Check sheet for the modelled part. Datum: model origin and axes. Units: mm. A direction names the side the tool comes from. Round coordinates to 2 decimals unless told otherwise and drop trailing zeros. Order: outer loops, then holes, each group sorted by start corner. A loop starts at its lowest first (then second) coordinate and runs counter-clockwise, first axis right, second up. Notation, with made-up numbers: (22, 28.5) -> (63, 28.5) arc R14 ccw to (63, 41.5) -> close; hole circle Ø1 at (2.5, 70.25). An arc over 180 degrees is marked (long way). Answer as CSV lines item,"result". Start each with the question number.
from build123d import *

# Parameters (mm, degrees)
SM_BASE_FLANGE_1_DEPTH = 2
OTHER_START            = -4.5
OTHER_3_DEPTH          = 20
OTHER_3_2_OUTLINE_W    = 2
OTHER_3_2_OUTLINE_H    = 24
OTHER_3_2_DEPTH        = 20
OTHER_START_2          = 5.5
OTHER_3_3_OUTLINE_W    = 2
OTHER_3_3_OUTLINE_H    = 15
OTHER_3_3_OUTLINE_H_2  = 9
OTHER_3_3_DEPTH        = 10
OTHER_START_3          = 4.5
OTHER_3_4_OUTLINE_W    = 2
OTHER_3_4_OUTLINE_H    = 15
OTHER_3_4_DEPTH        = 1
OTHER_4_DEPTH          = 20
OTHER_4_2_DEPTH        = 9
OTHER_4_3_DEPTH        = 11
OTHER_4_4_DEPTH        = 9
SKETCH_10_R            = 1.6
CUT_EXTRUDE_1_DEPTH    = 10
SKETCH_11_R            = 1.6
CUT_EXTRUDE_2_DEPTH    = 10
SKETCH_13_R            = 1.6
CUT_EXTRUDE_3_DEPTH    = 87
CUT_EXTRUDE_4_DEPTH    = 87
SKETCH_15_R            = 1.6
CUT_EXTRUDE_5_DEPTH    = 87
FILLET_1_R             = 3
FILLET_2_R             = 2


# Read off the part's stored shape, not the designer's step: 绘制的折弯3, 绘制的折弯4
# Sheet-metal steps are written as plain solids
with BuildPart() as part:
    # Sketch 1 → 基体-法兰1 (new body)
    with BuildSketch(Plane(origin=(0, 0, 0), x_dir=(1, 0, 0), z_dir=(0, 1, 0))):
        Polygon((-16, -15.5), (16, -15.5), (73, -15.5), (73, -4.5), (58, -4.5), (58, 4.5), (34, 4.5), (34, -5.5), (25, -5.5), (25, 4.5), (16, 4.5), (16, 15.5), (-16, 15.5), align=None)
    extrude(amount=-SM_BASE_FLANGE_1_DEPTH)

    # Other 3 outline → Other 3 (cut)
    with BuildSketch(Plane.XY.offset(OTHER_START)):
        with BuildLine():
            ThreePointArc((18.929203673, 0), (20.661254481, -0.550510257), (21.757630798, -2))
            Line((21.757630798, -2), (73, -2))
            Line((73, -2), (73, 0))
            Line((73, 0), (18.929203673, 0))
        make_face()
    extrude(amount=OTHER_3_DEPTH, mode=Mode.SUBTRACT)

    # Other 3 2 outline → Other 3 2 (add)
    with BuildSketch(Plane.XY.offset(OTHER_START)):
        with Locations((20.929203673, -26.929203673)):
            Rectangle(OTHER_3_2_OUTLINE_W, OTHER_3_2_OUTLINE_H)
        with BuildLine():
            Line((19.929203673, -3), (19.929203673, -5.929203673))
            Line((19.929203673, -5.929203673), (21.929203673, -5.929203673))
            Line((21.929203673, -5.929203673), (21.929203673, -3))
            ThreePointArc((21.929203673, -3), (21.885999352, -2.492694064), (21.757630798, -2))
            Line((21.757630798, -2), (18.929203673, -2))
            ThreePointArc((18.929203673, -2), (19.636310454, -2.292893219), (19.929203673, -3))
        make_face()
    extrude(amount=OTHER_3_2_DEPTH)

    # Other 3 3 outline → Other 3 3 (add)
    with BuildSketch(Plane.XY.offset(OTHER_START_2)):
        with Locations((20.929203673, -46.429203673)):
            Rectangle(OTHER_3_3_OUTLINE_W, OTHER_3_3_OUTLINE_H)
        with Locations((20.929203673, -10.429203673)):
            Rectangle(OTHER_3_3_OUTLINE_W, OTHER_3_3_OUTLINE_H_2)
    extrude(amount=OTHER_3_3_DEPTH)

    # Other 3 4 outline → Other 3 4 (add)
    with BuildSketch(Plane.XY.offset(OTHER_START_3)):
        with Locations((20.929203673, -46.429203673)):
            Rectangle(OTHER_3_4_OUTLINE_W, OTHER_3_4_OUTLINE_H)
    extrude(amount=OTHER_3_4_DEPTH)

    # Other 4 outline → Other 4 (cut)
    with BuildSketch(Plane.XY.offset(OTHER_START)):
        with BuildLine():
            Line((19.929203673, -40.186834471), (19.929203673, -53.929203673))
            Line((19.929203673, -53.929203673), (21.929203673, -53.929203673))
            Line((21.929203673, -53.929203673), (21.929203673, -37.358407346))
            ThreePointArc((21.929203673, -37.358407346), (21.378693416, -39.090458154), (19.929203673, -40.186834471))
        make_face()
    extrude(amount=OTHER_4_DEPTH, mode=Mode.SUBTRACT)

    # Other 4 2 outline → Other 4 2 (cut)
    with BuildSketch(Plane.XY.offset(OTHER_START)):
        Polygon((19.929203673, -38.929203673), (20.5, -38.929203673), (19.929203673, -38.358407347), align=None)
    extrude(amount=OTHER_4_2_DEPTH, mode=Mode.SUBTRACT)

    # Other 4 3 outline → Other 4 3 (add)
    with BuildSketch(Plane.XY.offset(OTHER_START_3)):
        with BuildLine():
            ThreePointArc((18.929203673, -40.358407346), (19.436509609, -40.315203025), (19.929203673, -40.186834471))
            Line((19.929203673, -40.186834471), (19.929203673, -37.358407346))
            ThreePointArc((19.929203673, -37.358407346), (19.636310454, -38.065514128), (18.929203673, -38.358407346))
            Line((18.929203673, -38.358407346), (5.5, -38.358407346))
            Line((5.5, -38.358407346), (5.5, -40.358407346))
            Line((5.5, -40.358407346), (18.929203673, -40.358407346))
        make_face()
    extrude(amount=OTHER_4_3_DEPTH)

    # Other 4 4 outline → Other 4 4 (add)
    with BuildSketch(Plane.XY.offset(OTHER_START)):
        with BuildLine():
            Line((20.5, -38.929203673), (21.050524017, -39.47972769))
            ThreePointArc((21.050524017, -39.47972769), (21.283955222, -39.217209419), (21.485098605, -38.929203673))
            Line((21.485098605, -38.929203673), (20.5, -38.929203673))
        make_face()
        with BuildLine():
            Line((19.636310454, -38.065514128), (19.929203673, -38.358407347))
            Line((19.929203673, -38.358407347), (19.929203673, -37.358407346))
            ThreePointArc((19.929203673, -37.358407346), (19.853083206, -37.741090779), (19.636310454, -38.065514128))
        make_face()
    extrude(amount=OTHER_4_4_DEPTH)

    # 草图10 → 切除-拉伸1 (cut)
    with BuildSketch(Plane(origin=(0, 0, 0), x_dir=(1, 0, 0), z_dir=(0, 1, 0))):
        with Locations(Location((-12.5, 12.5, 0), (0, 0, 270))):
            Circle(SKETCH_10_R)
        with Locations(Location((12.5, 12.5, 0), (0, 0, 270))):
            Circle(SKETCH_10_R)
    extrude(amount=-CUT_EXTRUDE_1_DEPTH, mode=Mode.SUBTRACT)

    # 草图11 → 切除-拉伸2 (cut)
    with BuildSketch(Plane(origin=(0, 0, 0), x_dir=(1, 0, 0), z_dir=(0, 1, 0))):
        with Locations(Location((-12.8, -12.3, 0), (0, 0, 270))):
            Circle(SKETCH_11_R)
        with Locations(Location((-4.5, -12.3, 0), (0, 0, 270))):
            Circle(SKETCH_11_R)
    extrude(amount=-CUT_EXTRUDE_2_DEPTH, mode=Mode.SUBTRACT)

    # 草图13 → 切除-拉伸3 (cut)
    with BuildSketch(Plane(origin=(0, -40.358407346, 0), x_dir=(-1, 0, 0), z_dir=(0, -1, 0))):
        with Locations(Location((-8.5, -10, 0), (0, 0, 180))):
            Circle(SKETCH_13_R)
        with Locations(Location((-15.5, -10, 0), (0, 0, 180))):
            Circle(SKETCH_13_R)
    extrude(amount=-CUT_EXTRUDE_3_DEPTH, mode=Mode.SUBTRACT)

    # 草图14 → 切除-拉伸4 (cut)
    with BuildSketch(Plane(origin=(21.929203673, 0, 0), x_dir=(0, 0, -1), z_dir=(1, 0, 0))):
        with BuildLine():
            Line((-10.3, -19.758407346), (-10.3, -20.179203673))
            Line((-10.3, -20.179203673), (-10.3, -21.358407346))
            ThreePointArc((-10.3, -21.358407346), (-9.16862915, -20.889778196), (-8.7, -19.758407346))
            ThreePointArc((-8.7, -19.758407346), (-9.16862915, -18.627036497), (-10.3, -18.158407346))
            Line((-10.3, -18.158407346), (-10.3, -19.758407346))
        make_face()
        with BuildLine():
            ThreePointArc((-10.3, -18.158407346), (-11.571470433, -18.78713862), (-11.843674335, -20.179203673))
            Line((-11.843674335, -20.179203673), (-10.3, -20.179203673))
            Line((-10.3, -20.179203673), (-10.3, -19.758407346))
            Line((-10.3, -19.758407346), (-10.3, -18.158407346))
        make_face()
        with BuildLine():
            Line((-10.3, -20.179203673), (-11.843674335, -20.179203673))
            ThreePointArc((-11.843674335, -20.179203673), (-11.271268726, -21.029877779), (-10.3, -21.358407346))
            Line((-10.3, -21.358407346), (-10.3, -20.179203673))
        make_face()
        with BuildLine():
            ThreePointArc((-8.7, -28.758407346), (-9.16862915, -27.627036497), (-10.3, -27.158407346))
            Line((-10.3, -27.158407346), (-10.3, -28.758407346))
            Line((-10.3, -28.758407346), (-10.3, -30.358407346))
            ThreePointArc((-10.3, -30.358407346), (-9.16862915, -29.889778196), (-8.7, -28.758407346))
        make_face()
        with BuildLine():
            Line((-10.3, -28.758407346), (-10.3, -27.158407346))
            ThreePointArc((-10.3, -27.158407346), (-11.9, -28.758407346), (-10.3, -30.358407346))
            Line((-10.3, -30.358407346), (-10.3, -28.758407346))
        make_face()
        with BuildLine():
            ThreePointArc((-8.7, -10.758407346), (-11.43137085, -9.627036497), (-10.3, -12.358407346))
            ThreePointArc((-10.3, -12.358407346), (-9.16862915, -11.889778196), (-8.7, -10.758407346))
        make_face()
    extrude(amount=-CUT_EXTRUDE_4_DEPTH, mode=Mode.SUBTRACT)

    # 草图15 → 切除-拉伸5 (cut)
    with BuildSketch(Plane(origin=(21.929203673, 0, 0), x_dir=(0, 0, -1), z_dir=(1, 0, 0))):
        with Locations(Location((-0.3, -28.758407346, 0), (0, 0, 90))):
            Circle(SKETCH_15_R)
    extrude(amount=-CUT_EXTRUDE_5_DEPTH, mode=Mode.SUBTRACT)

    # 圆角1
    fillet_1_edges = [part.edges().sort_by_distance(p)[0] for p in [
        (5.5, -39.358407346, 4.5),
        (5.5, -39.358407346, 15.5),
        (20.929203673, -5.929203673, -4.5),
        (20.929203673, -14.929203673, -4.5),
        (16, -1, -15.5),
        (-16, -1, -15.5),
        (-16, -1, 15.5),
    ]]
    fillet(fillet_1_edges, radius=FILLET_1_R)

    # 圆角2
    fillet_2_edges = [part.edges().sort_by_distance(p)[0] for p in [
        (20.929203673, -5.929203673, 5.5),
        (20.929203673, -14.929203673, 5.5),
    ]]
    fillet(fillet_2_edges, radius=FILLET_2_R)


solid = part.part
1) Section check C-C on y = -32.5. Record the cut outline in (x, z).
2) Mould release check, pull along Y, two halves, no side actions. Record for faces 1 (the face through (20.943, -15.831, -3.645)), 2 (the face through (12, -40.358, 10)), 3 (the face through (0, -1, -15.5)): released by +Y, released by -Y, zero draft, split by the parting line, or undercut.
3) Section check D-D on z = -7. Record the cut outline in (x, y).
4) Section check A-A on x = -4.5. Record the cut outline in (y, z).
5) Access from +Z, -Z, +X, -X, +Y, -Y to the whole of each face (thin tool, end or side, straight path). Record for faces 4 (the face through (20.9, -6.5, 4.9)), 5 (the face through (21.929, -20, 5)), 6 (the face through (19, -1, -4.5)), 7 (the face through (5.5, -39, 10)), 8 (the face through (19.628, -2.285, 5.36)).
6) Material ranges on line 1 along Y through (x, z) = (6, 11.5); line 2 along Y through (x, z) = (-12.5, 9); line 3 along Z through (x, y) = (15.5, -39.7), recorded low to high.
7) Depth check by flat-ended pin: pin 1 Ø0.6 at (x, z) = (20.5, 0) entering from -Y; pin 2 Ø12 at (x, y) = (-5, -33) entering from -Z; pin 3 Ø5 at (x, z) = (12.5, -12.5) entering from +Y; pin 4 Ø4 at (x, z) = (-12.5, -12.5) entering from -Y. Enter the tip coordinate at first touch or a pass-through.
8) Section check B-B on z = -0.5. Record the cut outline in (x, y).
Solutions:
1,outline,"(19.93, -4.5) -> (21.93, -4.5) -> (21.93, 15.5) -> (19.93, 15.5) -> close"
2,face 1,"undercut"
2,face 2,"released by -Y"
2,face 3,"zero draft"
3,outline,"(-16, -2) -> (16, -2) -> (16, 0) -> (-16, 0) -> close"
4,outline,"(-2, -15.5) -> (0, -15.5) -> (0, 10.7) -> (-2, 10.7) -> close; (-2, 13.9) -> (0, 13.9) -> (0, 15.5) -> (-2, 15.5) -> close"
5,face 4,"-Z, +X, -X"
5,face 5,"+Z, -Z, +X, +Y, -Y"
5,face 6,"-Z, +X, +Y, -Y"
5,face 7,"+Z, -Z, -X, -Y"
5,face 8,"+Z, -Z, -X"
6,line 1,"y = -40.36 to -38.36, -2 to 0"
6,line 2,"y = -2 to 0"
6,line 3,"z = 4.5 to 8.4, 11.6 to 15.5"
7,pin 1,"stops at y = -39.23"
7,pin 2,"passes through"
7,pin 3,"stops at y = 0"
7,pin 4,"stops at y = -2"
8,outline,"(-16, -2) -> (18.93, -2) arc R1 cw to (19.93, -3) -> (19.93, -5.93) -> (21.93, -5.93) -> (21.93, -3) arc R3 ccw to (18.93, 0) -> (-16, 0) -> close; (19.64, -38.07) -> (21.05, -39.48) arc R3 ccw to (21.93, -37.36) -> (21.93, -30.14) -> (19.93, -30.14) -> (19.93, -37.36) arc R1 cw to start; (19.93, -27.37) -> (21.93, -27.37) -> (21.93, -14.93) -> (19.93, -14.93) -> close"
